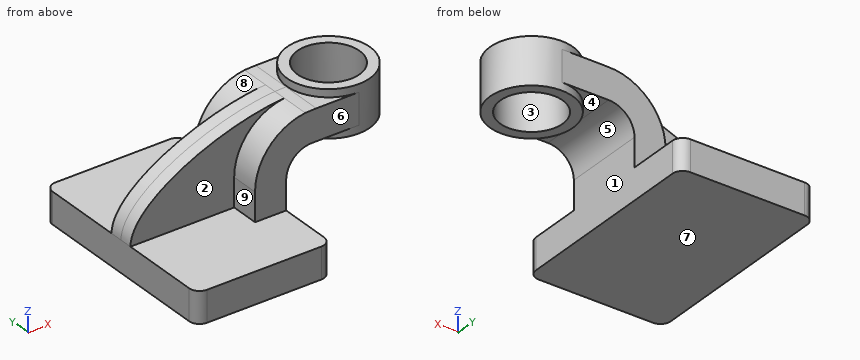
from build123d import *

# Parameters (mm, degrees)
F1_DEPTH = 63.5
F0_W     = 25.4
F0_H     = 19.05
F2_DEPTH = 25.4
F3_DEPTH = 7.9375
F5_R     = 6.35
F6_R     = 19.05
F7_DEPTH = 28.575


with BuildPart() as f1:
    # F0 (on Front) → F1 (new body, symmetric)
    with BuildSketch(Plane.XZ):
        Polygon((22.225, 9.525), (-41.275, 9.525), (-41.275, -9.525), (41.275, -9.525), (41.275, 9.525), align=None)
    extrude(amount=F1_DEPTH, both=True)

    # F0 (on Front) → F2 (join, symmetric)
    with BuildSketch(Plane.XZ):
        with BuildLine():
            Line((22.225, 27.0002), (22.225, 9.525))
            Line((22.225, 9.525), (41.275, 9.525))
            Line((41.275, 9.525), (41.275, 27.0002))
            ThreePointArc((41.275, 27.0002), (45.9246798487, 38.2255201513), (57.15, 42.8752))
            Line((57.15, 42.8752), (60.325, 42.8752))
            Line((60.325, 42.8752), (60.325, 61.9252))
            Line((60.325, 61.9252), (59.6934049136, 61.9252))
            add(Edge.make_bspline(
                [(52.9561563715, 61.6724843294), (55.2525673411, 61.8319540941), (57.5026044371, 61.9176558632), (59.6934049136, 61.9252)],
                knots=[107.5361075689, 107.5361075689, 107.5361075689, 107.5361075689, 113.7209316461, 113.7209316461, 113.7209316461, 113.7209316461], degree=3))
            ThreePointArc((52.9561563715, 61.6724843294), (31.013573181, 50.165752403), (22.225, 27.0002))
        make_face()
        with Locations((73.025, 52.4002)):
            Rectangle(F0_W, F0_H)
    extrude(amount=F2_DEPTH, both=True)

    # F0 (on Front) → F3 (join, symmetric)
    with BuildSketch(Plane.XZ):
        with BuildLine():
            add(Edge.make_bspline(
                [(-41.275, 9.525), (-40.9189941995, 33.8261781517), (13.0282467061, 58.8997687996), (52.9561563715, 61.6724843294)],
                knots=[0, 0, 0, 0, 107.5361075689, 107.5361075689, 107.5361075689, 107.5361075689], degree=3))
            Line((-41.275, 9.525), (22.225, 9.525))
            Line((22.225, 9.525), (22.225, 27.0002))
            ThreePointArc((22.225, 27.0002), (31.013573181, 50.165752403), (52.9561563715, 61.6724843294))
        make_face()
    extrude(amount=F3_DEPTH, both=True)

    # F0 (on Front) → F4 (revolve)
    with BuildSketch(Plane.XZ):
        Polygon((85.725, 66.675), (85.725, 61.9252), (85.725, 42.8752), (85.725, 38.1), (111.125, 38.1), (111.125, 66.675), align=None)
    revolve(axis=Axis((85.725, 0, 52.3875), (0, 0, 1)))

    # F5
    f5_edges = [f1.edges().sort_by_distance(p)[0] for p in [
        (41.275, -63.5, 0),
        (-41.275, -63.5, 0),
        (41.275, 63.5, 0),
        (-41.275, 63.5, 0),
    ]]
    fillet(f5_edges, radius=F5_R)

    # F6 (on face) → F7 (cut, through all)
    with BuildSketch(Plane.XY.offset(66.675)):
        with Locations((85.725, 0)):
            Circle(F6_R)
    extrude(amount=-F7_DEPTH, mode=Mode.SUBTRACT)


solid = f1.part
Design review of the part built by this model. Coordinates are the model's own, in mm. Face numbers are marked on the shaded views. A direction names the side the tool comes from. Round coordinates to 2 decimals unless told otherwise and drop trailing zeros. Write each loop counter-clockwise with the first axis right and the second up, starting at its lowest first coordinate (ties: lowest second). Pieces come first, ordered by that corner, then holes. Notation, with made-up numbers: (1, 7.25) - (51, 7.25) arc R18 cw to (51, 33.25) - close; hole circle Ø5 at (31, 77.5). An arc over 180 degrees is marked (long way). Use a Markdown table: item, result. Add a question column.
1. Mouldability with a two-part tool opening along X and no side actions: class the marked faces 1, 2, 3 and 4 as +X half, -X half, draft (parallel to the pull), parting line (faces both ways), or undercut.
2. We need section A-A (x = 90.5). State the section outline as (y, z) points (3 decimals).
3. For the marked faces 5, 6, 7, 8 and 9, list the 3-axis set-ups (+Z, -Z, +X, -X, +Y, -Y) from which the entire face can be reached by the end or side of a thin tool; tool diameter is ignored.
4. Clearance check with flat-ended pins moving along their axes: pin 1 (1 mm diameter, centred on x = 12.5, y = 25, fed in from +Z) (3 decimals); pin 2 (10 mm diameter, centred on x = -15, z = 21.5, fed in from +Y); pin 3 (18.5 mm diameter, centred on y = 3.5, z = 8.5, fed in from +X) (3 decimals); pin 4 (12 mm diameter, centred on y = 37, z = 25.5, fed in from +X). State where each tip first meets the part, or that it passes through.
5. We need section B-B (y = -47). State the section outline as (x, z) points (3 decimals), then the cut area to 3 significant figures.
6. Wall thickness on probe 1 along X at (y, z) = (18.5, 7.5) (3 decimals); probe 2 along Y at (x, z) = (20, 47.5); probe 3 along Z at (x, y) = (-9, -12) (3 decimals): over which ranges is each line inside the solid? List them lowest first.
Output:
| question | item | result |
|---|---|---|
| 1 | face 1 | +X half |
| 1 | face 2 | draft |
| 1 | face 3 | undercut |
| 1 | face 4 | undercut |
| 2 | outline | (-24.947, 38.1) - (-18.442, 38.1) - (-18.442, 66.675) - (-24.947, 66.675) - close; (18.442, 38.1) - (24.947, 38.1) - (24.947, 66.675) - (18.442, 66.675) - close |
| 3 | face 5 | -Z, +Y, -Y |
| 3 | face 6 | +Z, +X, -X, -Y |
| 3 | face 7 | -Z, +X, -X, +Y, -Y |
| 3 | face 8 | +Z, -X, +Y |
| 3 | face 9 | +Z, -X, -Y |
| 4 | pin 1 | stops at z = 9.525 |
| 4 | pin 2 | stops at y = 7.94 |
| 4 | pin 3 | stops at x = 41.275 |
| 4 | pin 4 | passes through |
| 5 | outline | (-41.275, -9.525) - (41.275, -9.525) - (41.275, 9.525) - (-41.275, 9.525) - close |
| 5 | area | 1,570 mm2 |
| 6 | probe 1 | x = -41.275 to 41.275 |
| 6 | probe 2 | y = -7.94 to 7.94 |
| 6 | probe 3 | z = -9.525 to 9.525 |
